Read the model definition and answer for the solid it produces. Units are mm, in the model's axes. Face numbers are marked on the shaded views. A direction names the side the tool comes from. Give positions to 0.01 mm unless a question says otherwise; leave off trailing zeros. Write each loop counter-clockwise with the first axis right and the second up, starting at its lowest first coordinate (ties: lowest second). Pieces come first, ordered by that corner, then holes.
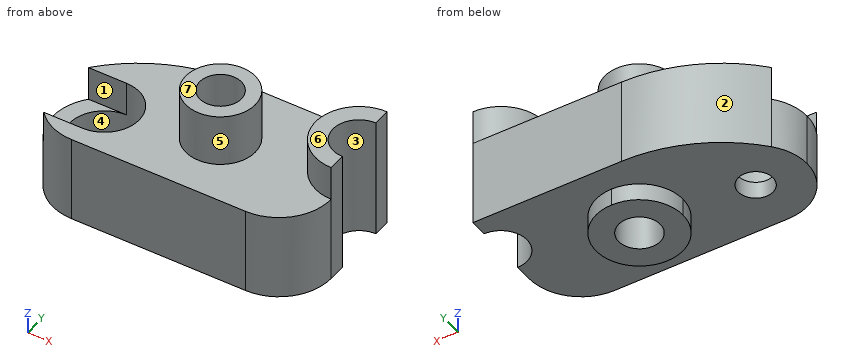
```python
from build123d import *

# Parameters (mm, degrees)
SKETCH1_W           = 160
SKETCH1_H           = 80
BOSS_EXTRUDE1_DEPTH = 90
CUT_EXTRUDE1_DEPTH  = 90
CUT_EXTRUDE2_DEPTH  = 90
SKETCH4_W           = 10
SKETCH4_H           = 15
CUT_EXTRUDE3_DEPTH  = 215
CUT_EXTRUDE4_DEPTH  = 10
CUT_EXTRUDE6_DEPTH  = 263
SKETCH7_W           = 160
SKETCH7_H           = 80
CUT_EXTRUDE7_DEPTH  = 263
SKETCH8_R           = 20
BOSS_EXTRUDE2_DEPTH = 30
SKETCH9_R           = 11
CUT_EXTRUDE8_DEPTH  = 117
BOSS_EXTRUDE3_DEPTH = 20
CUT_EXTRUDE9_DEPTH  = 20
SKETCH12_R          = 20
CUT_EXTRUDE10_DEPTH = 40
SKETCH13_R          = 10
CUT_EXTRUDE11_DEPTH = 40
SKETCH14_R          = 12
CUT_EXTRUDE12_DEPTH = 114


with BuildPart() as part:
    # Sketch1 → Boss-Extrude1 (new body)
    with BuildSketch(Plane.XY):
        with Locations((80, 40)):
            Rectangle(SKETCH1_W, SKETCH1_H)
    extrude(amount=BOSS_EXTRUDE1_DEPTH)

    # Sketch2 → Cut-Extrude1 (cut)
    with BuildSketch(Plane.XY.offset(90)):
        with BuildLine():
            ThreePointArc((160, 70), (145, 55), (160, 40))
            Line((160, 40), (160, 70))
        make_face()
        with BuildLine():
            ThreePointArc((160, 30), (151.213203436, 8.786796564), (130, 0))
            Line((130, 0), (160, 0))
            Line((160, 0), (160, 30))
        make_face()
    extrude(amount=-CUT_EXTRUDE1_DEPTH, mode=Mode.SUBTRACT)

    # Sketch3 → Cut-Extrude2 (cut)
    with BuildSketch(Plane.XY.offset(90)):
        with BuildLine():
            Line((0, 30), (0, 0))
            Line((0, 0), (30, 0))
            ThreePointArc((30, 0), (8.786796564, 8.786796564), (0, 30))
        make_face()
    extrude(amount=-CUT_EXTRUDE2_DEPTH, mode=Mode.SUBTRACT)

    # Sketch4 → Cut-Extrude3 (cut)
    with BuildSketch(Plane.ZY):
        with Locations((5, 72.5)):
            Rectangle(SKETCH4_W, SKETCH4_H)
        with Locations((5, 7.5)):
            Rectangle(SKETCH4_W, SKETCH4_H)
    extrude(amount=-CUT_EXTRUDE3_DEPTH, mode=Mode.SUBTRACT)

    # Sketch5 → Cut-Extrude4 (cut)
    with BuildSketch(Plane(origin=(0, 0, 0), x_dir=(-1, 0, 0), z_dir=(0, 0, -1))):
        with BuildLine():
            ThreePointArc((-90, 15), (-115, 40), (-90, 65))
            Line((-90, 65), (-148.819660113, 65))
            ThreePointArc((-148.819660113, 65), (-146.306936062, 48.876275643), (-160, 40))
            Line((-160, 40), (-160, 30))
            ThreePointArc((-160, 30), (-158.977774789, 22.235428647), (-155.980762114, 15))
            Line((-155.980762114, 15), (-90, 15))
        make_face()
        with BuildLine():
            Line((0, 65), (-90, 65))
            ThreePointArc((-90, 65), (-72.32233047, 57.67766953), (-65, 40))
            ThreePointArc((-65, 40), (-72.32233047, 22.32233047), (-90, 15))
            Line((-90, 15), (-4.019237886, 15))
            ThreePointArc((-4.019237886, 15), (-1.022225211, 22.235428647), (0, 30))
            Line((0, 30), (0, 65))
        make_face()
    extrude(amount=-CUT_EXTRUDE4_DEPTH, mode=Mode.SUBTRACT)

    # Sketch6 → Cut-Extrude6 (cut)
    with BuildSketch(Plane.XY.offset(90)):
        with BuildLine():
            Line((0, 30), (0, 80))
            Line((0, 80), (74.72135955, 80))
            ThreePointArc((74.72135955, 80), (37.979013408, 72.158383626), (7.639320225, 50))
            ThreePointArc((7.639320225, 50), (1.974829231, 40.704662693), (0, 30))
        make_face()
    extrude(amount=-CUT_EXTRUDE6_DEPTH, mode=Mode.SUBTRACT)

    # Sketch7 → Cut-Extrude7 (cut)
    with BuildSketch(Plane.XY.offset(60)):
        with Locations((80, 40)):
            Rectangle(SKETCH7_W, SKETCH7_H)
    extrude(amount=CUT_EXTRUDE7_DEPTH, mode=Mode.SUBTRACT)

    # Sketch8 → Boss-Extrude2 (add)
    with BuildSketch(Plane.XY.offset(60)):
        with Locations((90, 40)):
            Circle(SKETCH8_R)
    extrude(amount=BOSS_EXTRUDE2_DEPTH)

    # Sketch9 → Cut-Extrude8 (cut)
    with BuildSketch(Plane.XY.offset(90)):
        with Locations((90, 40)):
            Circle(SKETCH9_R)
    extrude(amount=-CUT_EXTRUDE8_DEPTH, mode=Mode.SUBTRACT)

    # Sketch10 → Boss-Extrude3 (add)
    with BuildSketch(Plane.XY.offset(60)):
        with BuildLine():
            Line((160, 40), (160, 30))
            ThreePointArc((160, 30), (135, 55), (160, 80))
            Line((160, 80), (160, 70))
            ThreePointArc((160, 70), (145, 55), (160, 40))
        make_face()
    extrude(amount=BOSS_EXTRUDE3_DEPTH)

    # Sketch11 → Cut-Extrude9 (cut)
    with BuildSketch(Plane.XY.offset(60)):
        with BuildLine():
            ThreePointArc((29.639320225, 10), (9.639320225, 30), (29.639320225, 50))
            Line((29.639320225, 50), (7.639320225, 50))
            ThreePointArc((7.639320225, 50), (0, 30), (7.639320225, 10))
            Line((7.639320225, 10), (29.639320225, 10))
        make_face()
    extrude(amount=-CUT_EXTRUDE9_DEPTH, mode=Mode.SUBTRACT)

    # Sketch12 → Cut-Extrude10 (cut)
    with BuildSketch(Plane.XY.offset(60)):
        with Locations((29.639320225, 30)):
            Circle(SKETCH12_R)
    extrude(amount=-CUT_EXTRUDE10_DEPTH, mode=Mode.SUBTRACT)

    # Sketch13 → Cut-Extrude11 (cut)
    with BuildSketch(Plane.XY.offset(20)):
        with Locations((29.639320225, 30)):
            Circle(SKETCH13_R)
    extrude(amount=-CUT_EXTRUDE11_DEPTH, mode=Mode.SUBTRACT)

    # Sketch14 → Cut-Extrude12 (cut)
    with BuildSketch(Plane.XY.offset(90)):
        with Locations((90, 40)):
            Circle(SKETCH14_R)
    extrude(amount=-CUT_EXTRUDE12_DEPTH, mode=Mode.SUBTRACT)


solid = part.part
```
Item 1: Section B-B (y = 42) is taken. Write down the section's boundary in (x, z), and give its area (3 significant figures).
Result set:
outline: (2.5, 10) - (65.08, 10) - (65.08, 0) - (78.17, 0) - (78.17, 90) - (70.1, 90) - (70.1, 60) - (45.64, 60) - (45.64, 20) - (13.64, 20) - (13.64, 40) - (2.5, 40) - close; (101.83, 0) - (114.92, 0) - (114.92, 10) - (152.52, 10) - (152.52, 80) - (138.65, 80) - (138.65, 60) - (109.9, 60) - (109.9, 90) - (101.83, 90) - close
area: 5,840 mm2
Item 2: Which of the six approach directions +Z, -Z, +X, -X, +Y, -Y give full straight-line access (tool end or side, diameter ignored) to the marked faces 5, 6 and 7?
Result set:
face 5: +Z
face 6: +Z, +X, +Y, -Y
face 7: +Z, +X, -X, +Y, -Y
Item 3: Find the intervals of material crossed by line 1 along X through (y, z) = (30, 33.5); line 2 along X through (y, z) = (48, 38); line 3 along Z through (x, y) = (47, 11.5), in increasing order.
Result set:
line 1: x = 0 to 9.64, 49.64 to 83.37, 96.63 to 160
line 2: x = 6 to 20.92, 38.36 to 81.06, 98.94 to 146.73
line 3: z = 10 to 60
Item 4: Each of these flat-tipped pins is pushed along its axis until it touches: pin 1 Ø1 at (y, z) = (10, 24.5) entering from +X; pin 2 Ø1.5 at (y, z) = (59, 79.5) entering from -X; pin 3 Ø24 at (x, y) = (47, 31.5) entering from +Z. Where does it stop, or does it pass through?
Result set:
pin 1: stops at x = 152.8
pin 2: stops at x = 81.82
pin 3: stops at z = 60
Item 5: Section A-A (z = 32) is taken. Write down the section's boundary in (x, y), and give its area (3 significant figures).
Result set:
outline: (7.64, 50) arc R30 ccw to (30, 0) - (130, 0) arc R30 ccw to (160, 30) - (160, 40) arc R15 cw to (160, 70) - (160, 80) - (74.72, 80) arc R90 ccw to start; hole circle Ø40 at (29.64, 30); hole circle Ø24 at (90, 40)
area: 9,460 mm2
Item 6: Section C-C (x = 93) is taken. Write down the section's boundary in (y, z), and give its area (3 significant figures).
Result set:
outline: (0, 10) - (15.18, 10) - (15.18, 0) - (28.38, 0) - (28.38, 90) - (20.23, 90) - (20.23, 60) - (0, 60) - close; (51.62, 0) - (64.82, 0) - (64.82, 10) - (80, 10) - (80, 60) - (59.77, 60) - (59.77, 90) - (51.62, 90) - close
area: 3,590 mm2
Item 7: Section D-D (z = 6.5) is taken. Write down the section's boundary in (x, y), and give its area (3 significant figures).
Result set:
outline: circle Ø50 at (90, 40); hole circle Ø24 at (90, 40)
area: 1,510 mm2
Item 8: Determine the mould class of the marked faces 1, 2, 3 and 4 for opening direction X: pulls with the +X half, pulls with the -X half, needs draft (parallel to the pull), parting line crosses it, or undercut.
Result set:
face 1: needs draft
face 2: pulls with the -X half
face 3: pulls with the +X half
face 4: undercut
